Could you check a few things on this model? Use its own coordinates, in mm. Round coordinates to 2 decimals unless told otherwise and drop trailing zeros. Write each loop counter-clockwise with the first axis right and the second up, starting at its lowest first coordinate (ties: lowest second). Pieces come first, ordered by that corner, then holes. Notation, with made-up numbers: (33.5, 34.25) -> (53.5, 34.25) arc R9 ccw to (53.5, 45.25) -> close; hole circle Ø4 at (49.5, 25.25). An arc over 180 degrees is marked (long way). Return JSON: item names as keys, results as strings.
from build123d import *

# Parameters (mm, degrees)
CROQUIS1_R              = 0.5
SALIENTE_EXTRUIR2_DEPTH = 0.2


with BuildPart() as part:
    # Croquis1 → Saliente-Extruir2 (new body)
    with BuildSketch(Plane.XY):
        with BuildLine():
            Line((-1.620168748, 13.5), (-0.633616905, 0.401284958))
            ThreePointArc((-0.633616905, 0.401284958), (0, -0.75), (0.633616905, 0.401284958))
            Line((0.633616905, 0.401284958), (1.620168748, 13.5))
            Line((1.620168748, 13.5), (0, 17.5))
            Line((0, 17.5), (-1.620168748, 13.5))
        make_face()
        Circle(CROQUIS1_R, mode=Mode.SUBTRACT)
    extrude(amount=SALIENTE_EXTRUIR2_DEPTH)


solid = part.part
1) I want a section at A-A, the plane y = 0. Please give me the cut outline in (x, z), and give its area (4 significant figures).
Return value:
{"outline": "(-0.75, 0) -> (-0.5, 0) -> (-0.5, 0.2) -> (-0.75, 0.2) -> close; (0.5, 0) -> (0.75, 0) -> (0.75, 0.2) -> (0.5, 0.2) -> close", "area": "0.1000 mm²"}
2) I want a section at C-C, the plane x = -1. Please give me the cut outline in (y, z), and give its area (3 significant figures).
Return value:
{"outline": "(5.27, 0) -> (15.03, 0) -> (15.03, 0.2) -> (5.27, 0.2) -> close", "area": "1.95 mm²"}
3) I want a section at D-D, the plane y = 15.25. Please give me the cut outline in (x, z).
Return value:
{"outline": "(-0.91, 0) -> (0.91, 0) -> (0.91, 0.2) -> (-0.91, 0.2) -> close"}
4) I want a section at B-B, the plane z = 0.15. Please give me the cut outline in (x, y).
Return value:
{"outline": "(-1.62, 13.5) -> (-0.63, 0.4) arc R0.75 ccw (long way) to (0.63, 0.4) -> (1.62, 13.5) -> (0, 17.5) -> close; hole circle Ø1 at (0, 0)"}
5) If I drill on probe 1 along Y at (x, z) = (-0.4, 0.1); probe 2 along X at (y, z) = (3.25, 0.1); probe 3 along X at (y, z) = (10, 0.15), over which ranges is the centre line in solid material (lowest first)? Write a range as [from, to].
Return value:
{"probe 1": "[-0.63, -0.3], [0.3, 16.51]", "probe 2": "[-0.85, 0.85]", "probe 3": "[-1.36, 1.36]"}
